Could you check a few things on this drawing? It's one solid part, dimensions in mm from its lowest x, y, z. Round coordinates to 2 decimals unless told otherwise and drop trailing zeros. Loops run counter-clockwise (first coordinate to the right, second up) from the corner with the lowest first, then second, coordinate; pieces in that order, holes last. Notation, with made-up numbers: (88.25, -14) -> (99.25, -14) arc R12 ccw to (99.25, -5) -> close; hole circle Ø9 at (10.25, -37). An arc over 180 degrees is marked (long way). Write each question's results on one line, items separated by ' | '.
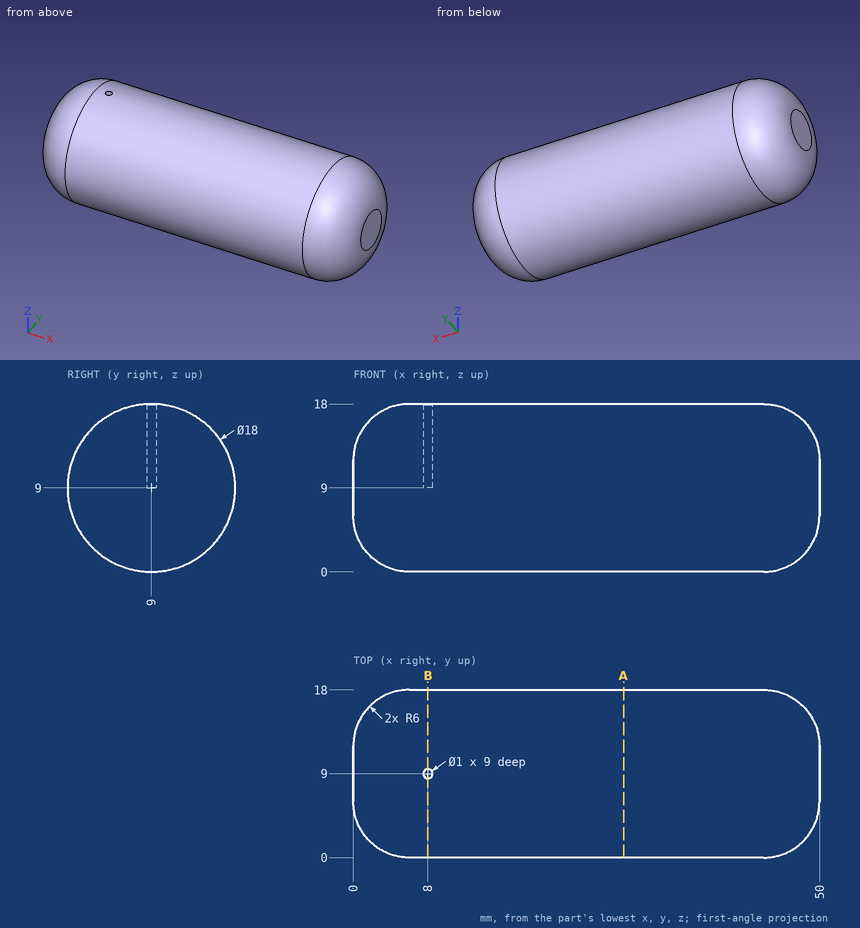
1) I'm going to push flat-ended pins straight in: pin 1 (6 mm diameter, centred on y = 15, z = 15.5, fed in from -X); pin 2 (5 mm diameter, centred on x = 16, y = 6, fed in from -Z); pin 3 (1.5 mm diameter, centred on x = 32, y = 13, fed in from -Z). Where does each tip first touch, or does it pass through?
Model answer:
pin 1: stops at x = 0.72 | pin 2: stops at z = 0.01 | pin 3: stops at z = 0.61
2) I want a section at A-A, the plane x = 29. Write out the boundary of the cut face in (y, z).
Model answer:
outline: circle Ø18 at (9, 9)
3) I want a section at B-B, the plane x = 8. Write out the boundary of the cut face in (y, z), plus the area to 3 significant figures.
Model answer:
outline: (8.5, 9) -> (8.5, 17.99) arc R9 ccw (long way) to (9.5, 17.99) -> (9.5, 9) -> close | area: 245 mm2
4) I need wall thicknesses on line 1 (Y direction, x = 8, z = 11.5); line 2 (Y direction, x = 8, z = 15.75); line 3 (Z direction, x = 25.5, y = 9.25). Which ranges of each line are inside material? Lowest first, please.
Model answer:
line 1: y = 0.35 to 8.5, 9.5 to 17.65 | line 2: y = 3.05 to 8.5, 9.5 to 14.95 | line 3: z = 0 to 18
